The model under review builds one solid part; all positions refer to its coordinate system, in mm. Face numbers are marked on the shaded views. A direction names the side the tool comes from. Coordinates: 2 decimals unless noted, no trailing zeros. Order: outer loops, then holes, each group sorted by start corner. A loop starts at its lowest first (then second) coordinate and runs counter-clockwise, first axis right, second up. Notation, with made-up numbers: M 8,-10.75 L 62,-10.75 A9 cw 62,4.25 Z; hole C 45,-6 d8. An arc over 180 degrees is marked long. Write each question's results on one line, items separated by ' | '.
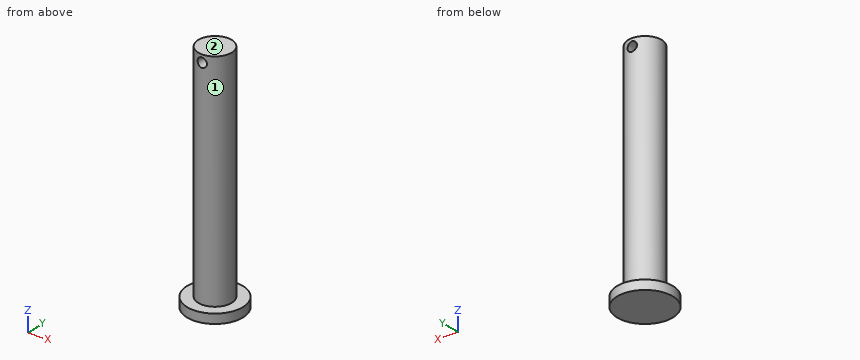
from build123d import *

# Parameters (mm, degrees)
F0_R     = 9
F1_DEPTH = 125
F2_R     = 15
F3_DEPTH = 5
F4_R     = 2.5
F5_DEPTH = 12.5


with BuildPart() as f1:
    # F0 (on Top) → F1 (new body)
    with BuildSketch(Plane.XY):
        Circle(F0_R)
    extrude(amount=F1_DEPTH)

    # F2 (on Top) → F3 (join)
    with BuildSketch(Plane.XY):
        Circle(F2_R)
    extrude(amount=F3_DEPTH)

    # F4 (on Front) → F5 (cut, symmetric)
    with BuildSketch(Plane.XZ):
        with Locations((0, 121)):
            Circle(F4_R)
    extrude(amount=F5_DEPTH, both=True, mode=Mode.SUBTRACT)


solid = f1.part
1) For the marked faces 1 and 2, list the 3-axis set-ups (+Z, -Z, +X, -X, +Y, -Y) from which the entire face can be reached by the end or side of a thin tool; tool diameter is ignored.
Solutions:
face 1: +Z | face 2: +Z, +X, -X, +Y, -Y
2) Take a section at A-A on y = 0. State the section outline as (x, z) points.
Solutions:
outline: M -15,0 L 15,0 L 15,5 L 9,5 L 9,125 L -9,125 L -9,5 L -15,5 Z; hole C 0,121 d5
3) For pin 1 (12 mm diameter, centred on x = -5, z = 25.5, fed in from +Y); pin 2 (3 mm diameter, centred on x = -7, z = 21, fed in from -Y); pin 3 (8 mm diameter, centred on y = 8, z = 54, fed in from +X); pin 4 (1.5 mm diameter, centred on x = 10.5, z = 71, fed in from -Y), all flat-tipped, find the tip position at first contact; note any pin that passes through.
Solutions:
pin 1: y = 9 | pin 2: y = -7.12 | pin 3: x = 8.06 | pin 4: through
4) To check wall thickness, follow line 1 along Z through (x, y) = (0, 1.25); line 2 along X through (y, z) = (0.5, 86); line 3 along X through (y, z) = (-4.5, 121). State the ranges of each line that lie inside material, in increasing order.
Solutions:
line 1: 0 to 118.5, 123.5 to 125 | line 2: -8.99 to 8.99 | line 3: -7.79 to -2.5, 2.5 to 7.79
5) Take a section at B-B on x = 0. State the section outline as (y, z) points, plus the area to 3 significant figures.
Solutions:
outline: M -15,0 L 15,0 L 15,5 L 9,5 L 9,118.5 L -9,118.5 L -9,5 L -15,5 Z; M -9,123.5 L 9,123.5 L 9,125 L -9,125 Z | area: 2,220 mm2
6) Take a section at D-D on x = -5.5. State the section outline as (y, z) points, plus the area to 3 significant figures.
Solutions:
outline: M -13.96,0 L 13.96,0 L 13.96,5 L 7.12,5 L 7.12,125 L -7.12,125 L -7.12,5 L -13.96,5 Z | area: 1,850 mm2
7) Take a section at C-C on z = 61.5. State the section outline as (x, y) points.
Solutions:
outline: C 0,0 d18
